Geometry: final body of the model. Coordinates: model frame, mm. Coordinates: 2 decimals unless noted, no trailing zeros. Write each loop counter-clockwise with the first axis right and the second up, starting at its lowest first coordinate (ties: lowest second). Pieces come first, ordered by that corner, then holes. Notation, with made-up numbers: (40.5, 12.25) -> (57.5, 12.25) arc R22 cw to (57.5, 25.25) -> close; hole circle Ø7 at (-12, -17.75). An arc over 180 degrees is marked (long way). One line per item, written item: value.
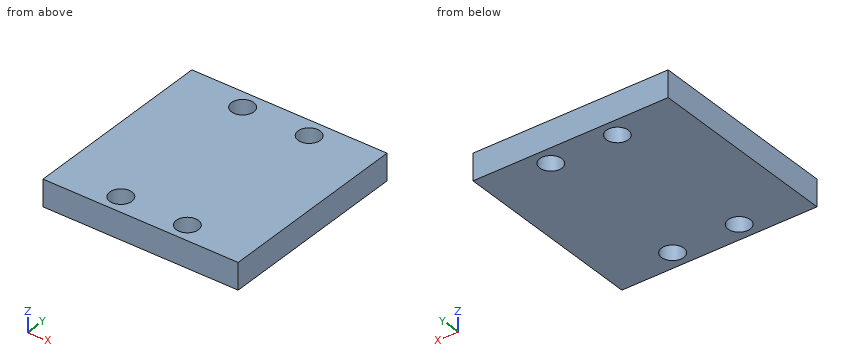
```python
from build123d import *

# Parameters (mm, degrees)
CYLINDER003_R     = 2.5
CYLINDER003_DEPTH = 10
CYLINDER002_R     = 2.5
CYLINDER002_DEPTH = 10
CYLINDER001_R     = 2.5
CYLINDER001_DEPTH = 10
CYLINDER_R        = 2.5
CYLINDER_DEPTH    = 10
BOX_W             = 44
BOX_H             = 44
BOX_DEPTH         = 6


with BuildPart() as cylinder003:
    # Cylinder003 → Cylinder003 (new body)
    with BuildSketch(Plane(origin=(29.5, 40, 0), x_dir=(1, 0, 0), z_dir=(0, 0, 1))):
        Circle(CYLINDER003_R)
    extrude(amount=CYLINDER003_DEPTH)


with BuildPart() as cylinder002:
    # Cylinder002 → Cylinder002 (new body)
    with BuildSketch(Plane(origin=(14.5, 40, 0), x_dir=(1, 0, 0), z_dir=(0, 0, 1))):
        Circle(CYLINDER002_R)
    extrude(amount=CYLINDER002_DEPTH)


with BuildPart() as cylinder001:
    # Cylinder001 → Cylinder001 (new body)
    with BuildSketch(Plane(origin=(29.5, 4, 0), x_dir=(1, 0, 0), z_dir=(0, 0, 1))):
        Circle(CYLINDER001_R)
    extrude(amount=CYLINDER001_DEPTH)


with BuildPart() as cylinder:
    # Cylinder → Cylinder (new body)
    with BuildSketch(Plane(origin=(14.5, 4, 0), x_dir=(1, 0, 0), z_dir=(0, 0, 1))):
        Circle(CYLINDER_R)
    extrude(amount=CYLINDER_DEPTH)


with BuildPart() as cut003:
    # Box → Box (new body)
    with BuildSketch(Plane.XY):
        with Locations((22, 22)):
            Rectangle(BOX_W, BOX_H)
    extrude(amount=BOX_DEPTH)

    # Cut: cut Cylinder
    add(cylinder.part, mode=Mode.SUBTRACT)

    # Cut001: cut Cylinder001
    add(cylinder001.part, mode=Mode.SUBTRACT)

    # Cut002: cut Cylinder002
    add(cylinder002.part, mode=Mode.SUBTRACT)

    # Cut003: cut Cylinder003
    add(cylinder003.part, mode=Mode.SUBTRACT)


solid = cut003.part
```
(1) First-contact query: pin 1 (8 mm diameter, centred on x = 37, y = 9, fed in from -Z). Flat tip, straight axial feed; report the tip coordinate or a pass-through.
Responses:
pin 1: stops at z = 0
(2) Section A-A (y = 4). Return the cut outline in (x, z), then the cut area to 3 significant figures.
Responses:
outline: (0, 0) -> (12, 0) -> (12, 6) -> (0, 6) -> close; (17, 0) -> (27, 0) -> (27, 6) -> (17, 6) -> close; (32, 0) -> (44, 0) -> (44, 6) -> (32, 6) -> close
area: 204 mm2
(3) Section C-C (z = 3.9). Return the cut outline in (x, y), then the cut area to 3 significant figures.
Responses:
outline: (0, 0) -> (44, 0) -> (44, 44) -> (0, 44) -> close; hole circle Ø5 at (14.5, 4); hole circle Ø5 at (14.5, 40); hole circle Ø5 at (29.5, 4); hole circle Ø5 at (29.5, 40)
area: 1,860 mm2
(4) Line query: line 1 (Y direction, x = 29.5, z = 2.75); line 2 (X direction, y = 4, z = 2.2); line 3 (X direction, y = 39, z = 1.4). Output: solid intervals per line, ascending. Write a range as [from, to].
Responses:
line 1: y = [0, 1.5], [6.5, 37.5], [42.5, 44]
line 2: x = [0, 12], [17, 27], [32, 44]
line 3: x = [0, 12.21], [16.79, 27.21], [31.79, 44]
(5) Section B-B (x = 14.5). Return the cut outline in (y, z), then the cut area to 3 significant figures.
Responses:
outline: (0, 0) -> (1.5, 0) -> (1.5, 6) -> (0, 6) -> close; (6.5, 0) -> (37.5, 0) -> (37.5, 6) -> (6.5, 6) -> close; (42.5, 0) -> (44, 0) -> (44, 6) -> (42.5, 6) -> close
area: 204 mm2
